Source: CAD feature listing. Evaluate the final solid. Frame: model axes, mm. Round coordinates to 2 decimals unless told otherwise and drop trailing zeros. Write each loop counter-clockwise with the first axis right and the second up, starting at its lowest first coordinate (ties: lowest second). Pieces come first, ordered by that corner, then holes. Notation, with made-up numbers: M 4,84 L 18,84 A29 cw 18,111 Z; hole C 88,60 d2. An arc over 180 degrees is marked long. Put each result on its own line as item: value. Start each with the question number.
```python
from build123d import *

# Parameters (mm, degrees)
CROQUIS1_W              = 290
CROQUIS1_H              = 330
SALIENTE_EXTRUIR1_DEPTH = 5


with BuildPart() as part:
    # Croquis1 → Saliente-Extruir1 (new body)
    with BuildSketch(Plane.XY):
        Polygon((-156.514277167, 244.450688952), (198.485722833, 244.450688952), (198.485722833, -105.549311048), (-161.514277167, -105.549311048), (-161.514277167, 234.450688952), (-156.514277167, 234.450688952), align=None)
        with Locations((-6.514277167, 69.450688952)):
            Rectangle(CROQUIS1_W, CROQUIS1_H, mode=Mode.SUBTRACT)
    extrude(amount=SALIENTE_EXTRUIR1_DEPTH)


solid = part.part
```
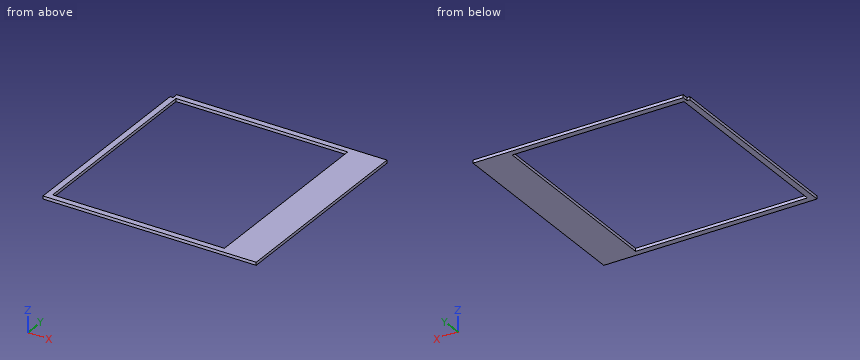
(1) Contact query for a flat-ended pin moving along its axis: P1, Ø2.5, axis at x = -159.5, z = 2.5, coming from the +Y side. Output: stop coordinate, or through.
(2) Section query A-A (x = 126). Return loops of the section in (y, z), and give its area (4 significant figures).
(3) Ray query, line 1 along Y through (x, z) = (122, 3.2); line 2 along X through (y, z) = (-34.5, 0.85). Return the intervals inside material, ascending.
(4) Section query C-C (z = 3.5). Return loops of the section in (x, y), and give its area (4 significant figures).
(5) Section query B-B (y = 1.5). Return loops of the section in (x, z).
Entries:
1. P1: y = 234.45
2. outline: M -105.55,0 L -95.55,0 L -95.55,5 L -105.55,5 Z; M 234.45,0 L 244.45,0 L 244.45,5 L 234.45,5 Z
2. area: 100.0 mm2
3. line 1: -105.55 to -95.55, 234.45 to 244.45
3. line 2: -161.51 to -151.51, 138.49 to 198.49
4. outline: M -161.51,-105.55 L 198.49,-105.55 L 198.49,244.45 L -156.51,244.45 L -156.51,234.45 L -161.51,234.45 Z; hole M -151.51,-95.55 L 138.49,-95.55 L 138.49,234.45 L -151.51,234.45 Z
4. area: 30,250 mm2
5. outline: M -161.51,0 L -151.51,0 L -151.51,5 L -161.51,5 Z; M 138.49,0 L 198.49,0 L 198.49,5 L 138.49,5 Z
